Geometry: final body of the model. Coordinates: model frame, mm. Face numbers are marked on the shaded views. A direction names the side the tool comes from. Give positions to 0.01 mm unless a question says otherwise; leave off trailing zeros. Loops run counter-clockwise (first coordinate to the right, second up) from the corner with the lowest first, then second, coordinate; pieces in that order, holes last. Notation, with made-up numbers: (48.5, -7.5) - (74.5, -7.5) arc R22 cw to (74.5, 21.5) - close; hole circle Ø5 at (-32, -18). An arc over 180 degrees is marked (long way). Use one line per item in the form item = value.
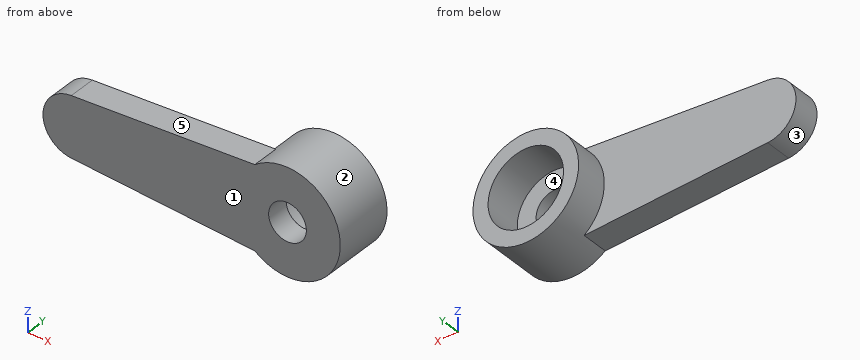
```python
from build123d import *

# Parameters (mm, degrees)
SKETCH1_R           = 3.5
SKETCH1_R_2         = 2.5
BOSS_EXTRUDE1_DEPTH = 4
BOSS_EXTRUDE2_DEPTH = 1.8
SKETCH3_R           = 2.5
SKETCH3_R_2         = 1.25
BOSS_EXTRUDE3_DEPTH = 1.5


with BuildPart() as part:
    # Sketch1 → Boss-Extrude1 (new body)
    with BuildSketch(Plane(origin=(0, 0, 0), x_dir=(1, 0, 0), z_dir=(0, 1, 0))):
        with Locations(Location((0, 0, 0), (0, 0, 270))):
            Circle(SKETCH1_R)
        with Locations(Location((0, 0, 0), (0, 0, 270))):
            Circle(SKETCH1_R_2, mode=Mode.SUBTRACT)
    extrude(amount=BOSS_EXTRUDE1_DEPTH)

    # Sketch2 → Boss-Extrude2 (add)
    with BuildSketch(Plane(origin=(0, 0, 0), x_dir=(1, 0, 0), z_dir=(0, 1, 0))):
        with BuildLine():
            Line((-2.165063509, 2.75), (-14.323761314, 1.996167112))
            ThreePointArc((-14.323761314, 1.996167112), (-16.2, 0), (-14.323761314, -1.996167112))
            Line((-14.323761314, -1.996167112), (-2.165063509, -2.75))
            ThreePointArc((-2.165063509, -2.75), (-3.5, 0), (-2.165063509, 2.75))
        make_face()
    extrude(amount=BOSS_EXTRUDE2_DEPTH)

    # Sketch3 → Boss-Extrude3 (add)
    with BuildSketch(Plane(origin=(0, 0, 0), x_dir=(1, 0, 0), z_dir=(0, 1, 0))):
        with Locations(Location((0, 0, 0), (0, 0, 270))):
            Circle(SKETCH3_R)
        with Locations(Location((0, 0, 0), (0, 0, 270))):
            Circle(SKETCH3_R_2, mode=Mode.SUBTRACT)
    extrude(amount=BOSS_EXTRUDE3_DEPTH)


solid = part.part
```
(1) Cut plane B-B (z = 0). Return the cut outline in (x, y).
Solution:
outline = (-16.2, 0) - (-1.25, 0) - (-1.25, 1.5) - (-2.5, 1.5) - (-2.5, 4) - (-3.5, 4) - (-3.5, 1.8) - (-16.2, 1.8) - close; (1.25, 0) - (3.5, 0) - (3.5, 4) - (2.5, 4) - (2.5, 1.5) - (1.25, 1.5) - close
(2) Pull-direction query (Z, two-part tool) for the marked faces 3, 4 and 5; classes: released by +Z, released by -Z, zero draft, split by the parting line, or undercut.
Solution:
face_3 = split by the parting line
face_4 = undercut
face_5 = released by +Z
(3) Cut plane D-D (z = 2.25). Return the cut outline in (x, y), plus the area to 3 significant figures.
Solution:
outline = (-10.23, 0) - (2.68, 0) - (2.68, 4) - (1.09, 4) - (1.09, 1.5) - (-1.09, 1.5) - (-1.09, 4) - (-2.68, 4) - (-2.68, 1.8) - (-10.23, 1.8) - close
area = 29.6 mm2
(4) Material intervals for L1, parallel to X at y = 3.15, z = 0; L2, parallel to Y at x = -8.75, z = -0.25; L3, parallel to X at y = 0.5, z = 0, sorted ascending. Write a range as from..to.
Solution:
L1 = -3.5..-2.5, 2.5..3.5
L2 = 0..1.8
L3 = -16.2..-1.25, 1.25..3.5
(5) Cut plane A-A (x = 0). Return the cut outline in (y, z).
Solution:
outline = (0, -3.5) - (4, -3.5) - (4, -2.5) - (1.5, -2.5) - (1.5, -1.25) - (0, -1.25) - close; (0, 1.25) - (1.5, 1.25) - (1.5, 2.5) - (4, 2.5) - (4, 3.5) - (0, 3.5) - close
(6) Pin query (flat end, axial travel): P1, Ø2, axis at y = 3.5, z = -3, coming from the +X side; P2, Ø1.6, axis at x = -8, z = 0, coming from the +Y side; P3, Ø1.5, axis at y = 2.5, z = 2, coming from the +X side; P4, Ø2, axis at x = 0, z = 0, coming from the -Y side. Return the tip coordinate at first contact, or that it passes through.
Solution:
P1 = 2.87
P2 = 1.8
P3 = 3.27
P4 = through
(7) Cut plane C-C (y = 2.75). Return the cut outline in (x, z), plus the area to 3 significant figures.
Solution:
outline = circle Ø7 at (0, 0); hole circle Ø5 at (0, 0)
area = 18.8 mm2
(8) Access query for the marked faces 1 and 2. Directions: +Z, -Z, +X, -X, +Y, -Y. A direction counts if a zero-diameter tool reaches every point of the face in a straight line with its end or side. Return the directions, or none.
Solution:
face_1 = +Z, -Z, +X, -X, -Y
face_2 = +Y
